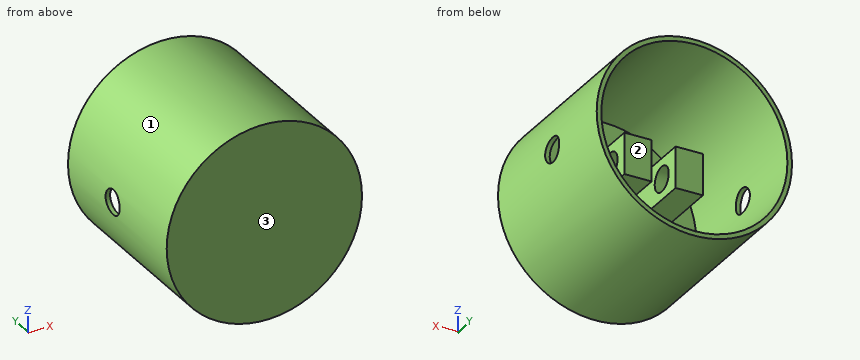
from build123d import *

# Parameters (mm, degrees)
F0_R     = 12.7
F1_DEPTH = 22.86
F2_R     = 12.102618
F3_DEPTH = 21.082
F5_DEPTH = 13.97
F6_R     = 1.6256
F7_DEPTH = 12.7


with BuildPart() as f1:
    # F0 (on Front) → F1 (new body)
    with BuildSketch(Plane.XZ):
        Circle(F0_R)
    extrude(amount=F1_DEPTH)

    # F2 (on face) → F3 (cut)
    with BuildSketch(Plane(origin=(0, 0, 0), x_dir=(-1, 0, 0), z_dir=(0, 1, 0))):
        Circle(F2_R)
    extrude(amount=-F3_DEPTH, mode=Mode.SUBTRACT)

    # F4 (on face) → F5 (join)
    with BuildSketch(Plane(origin=(0, -21.082, 0), x_dir=(-1, 0, 0), z_dir=(0, 1, 0))):
        Polygon((-1.553707, 2.682939), (-5.109707, 2.682939), (-5.109707, 0), (-5.109707, -2.682939), (-1.553707, -2.682939), (-1.553707, 0), align=None)
        Polygon((1.553707, 2.682939), (1.553707, 0), (1.553707, -2.682939), (5.109707, -2.682939), (5.109707, 0), (5.109707, 2.682939), align=None)
    extrude(amount=F5_DEPTH)

    # F6 (on Right) → F7 (cut, symmetric)
    with BuildSketch(Plane.YZ):
        with Locations((-10.320932, 0)):
            Circle(F6_R)
    extrude(amount=F7_DEPTH, both=True, mode=Mode.SUBTRACT)


solid = f1.part
CAD build for the part. Positions are in the model's coordinates, mm. Face numbers are marked on the shaded views. Round coordinates to 2 decimals unless told otherwise and drop trailing zeros. Write each loop counter-clockwise with the first axis right and the second up, starting at its lowest first coordinate (ties: lowest second). Pieces come first, ordered by that corner, then holes.
(1) Probe line 1 along Z through (x, y) = (0, -13); line 2 along Z through (x, y) = (3.5, -10); line 3 along Y through (x, z) = (11.5, -1). List the from-to ranges inside material, lowest first.
(2) Mould opens along Z. For the marked faces 1, 2 and 3 say: pulls with the +Z half, pulls with the -Z half, needs draft (parallel to the pull), parting line crosses it, or undercut.
(3) Slice it at D-D, the plane y = -9.25. Write the cut outline in (x, z), and give its area (3 significant figures).
(4) Slice it at A-A, the plane y = -14. Write the cut outline in (x, z).
(5) Slice it at C-C, the plane x = 0. Write the cut outline in (y, z).
(6) Drop flat-ended pins along their axis: P1, Ø6, axis at y = -13.5, z = -1, coming from the +X side; P2, Ø1.1, axis at x = 3.5, y = -15, coming from the +Z side; P3, Ø4, axis at x = -4, z = -0.5, coming from the +Y side; P4, Ø10, axis at y = -12.5, z = -7.5, coming from the +X side. Give the stop position or say it passes through.
(7) Slice it at B-B, the plane z = 0. Count the separate pieces of the cut face and the enclosed holes in it, and give its area (3 significant figures).
From the geometry:
1. line 1: z = -12.7 to -12.1, 12.1 to 12.7
1. line 2: z = -12.21 to -11.59, -2.68 to -1.59, 1.59 to 2.68, 11.59 to 12.21
1. line 3: y = -22.86 to -21.08
2. face 1: parting line crosses it
2. face 2: undercut
2. face 3: needs draft
3. outline: (-12.64, -1.22) arc R12.7 ccw to (12.64, -1.22) - (12.04, -1.22) arc R12.1 cw to (-12.04, -1.22) - close; (-12.64, 1.22) - (-12.04, 1.22) arc R12.1 cw to (12.04, 1.22) - (12.64, 1.22) arc R12.7 ccw to start; (-5.11, -2.68) - (-1.55, -2.68) - (-1.55, -1.22) - (-5.11, -1.22) - close; (-5.11, 1.22) - (-1.55, 1.22) - (-1.55, 2.68) - (-5.11, 2.68) - close; (1.55, -2.68) - (5.11, -2.68) - (5.11, -1.22) - (1.55, -1.22) - close; (1.55, 1.22) - (5.11, 1.22) - (5.11, 2.68) - (1.55, 2.68) - close
3. area: 64.4 mm2
4. outline: circle Ø25.4 at (0, 0); (-5.11, -2.68) - (-1.55, -2.68) - (-1.55, 2.68) - (-5.11, 2.68) - close; (1.55, -2.68) - (5.11, -2.68) - (5.11, 2.68) - (1.55, 2.68) - close; hole circle Ø24.21 at (0, 0)
5. outline: (-22.86, -12.7) - (0, -12.7) - (0, -12.1) - (-21.08, -12.1) - (-21.08, 12.1) - (0, 12.1) - (0, 12.7) - (-22.86, 12.7) - close
6. P1: stops at x = 12.7
6. P2: stops at z = 12.35
6. P3: stops at y = -7.11
6. P4: stops at x = 12.45
7. separate pieces: 5
7. enclosed holes: 0
7. area: 143 mm2
